```python
from build123d import *

# Parameters (mm, degrees)
F0_R     = 12.5
F1_DEPTH = 15


with BuildPart() as f1:
    # F0 (on Front) → F1 (new body)
    with BuildSketch(Plane.XZ):
        with BuildLine():
            ThreePointArc((-66.897273, -29.196363), (-41.384391, -23.525711), (-30, 0))
            ThreePointArc((-30, 0), (-41.384391, 23.525711), (-66.897273, 29.196363))
            ThreePointArc((-66.897273, 29.196363), (-90, 0), (-66.897273, -29.196363))
        make_face()
        with Locations((-60, 0)):
            Circle(F0_R, mode=Mode.SUBTRACT)
        with BuildLine():
            ThreePointArc((-66.897273, 29.196363), (-41.384391, 23.525711), (-30, 0))
            ThreePointArc((-30, 0), (-41.384391, -23.525711), (-66.897273, -29.196363))
            Line((-66.897273, -29.196363), (0, -45))
            Line((0, -45), (0, 45))
            Line((0, 45), (-66.897273, 29.196363))
        make_face()
    extrude(amount=F1_DEPTH)


solid = f1.part
```
CAD build for the part. Positions are in the model's coordinates, mm. Coordinates: 2 decimals unless noted, no trailing zeros. Write each loop counter-clockwise with the first axis right and the second up, starting at its lowest first coordinate (ties: lowest second). Pieces come first, ordered by that corner, then holes.
(1) Cut at A-A, the plane z = 0. List the corners of the cut face in (x, y).
(2) Flat gauge pins, fed straight in: pin 1 (6 mm diameter, centred on x = -30.5, y = -12, fed in from +Z); pin 2 (5 mm diameter, centred on x = -51.5, y = -3.5, fed in from +Z). Where does each tip first touch, or does it go through?
(3) Cut at C-C, the plane x = -60. List the corners of the cut face in (y, z), and give its area (3 significant figures).
(4) Two-plate mould, pull along Z, no slides. Class faces 1 (the face through (-72.488, -7.395, 0.55)), 2 (the face through (-33.917, -7.395, -36.988)), 3 (the face through (0, -7, -1)): +Z half, -Z half, draft (parallel to the pull), parting line (faces both ways), or undercut.
(5) Drill centre lines: probe 1 along Z at (x, y) = (-56.5, -10); probe 2 along X at (y, z) = (-1, -1); probe 3 along Z at (x, y) = (-60, -4.25). Where is each one in solid material? Low to high.
(6) Cut at B-B, the plane y = -6. List the corners of the cut face in (x, z).
(7) Cut at D-D, the plane x = -83. List the corners of the cut face in (y, z), and give its area (3 significant figures).
Geometry says:
1. outline: (-90, -15) - (-72.5, -15) - (-72.5, 0) - (-90, 0) - close; (-47.5, -15) - (0, -15) - (0, 0) - (-47.5, 0) - close
2. pin 1: stops at z = 38.5
2. pin 2: stops at z = 33.42
3. outline: (-15, -30.83) - (0, -30.83) - (0, -12.5) - (-15, -12.5) - close; (-15, 12.5) - (0, 12.5) - (0, 30.83) - (-15, 30.83) - close
3. area: 550 mm2
4. face 1: undercut
4. face 2: -Z half
4. face 3: draft
5. probe 1: z = -31.65 to -12, 12 to 31.65
5. probe 2: x = -89.98 to -72.46, -47.54 to 0
5. probe 3: z = -30.83 to -12.5, 12.5 to 30.83
6. outline: (-66.9, -29.2) - (0, -45) - (0, 45) - (-66.9, 29.2) arc R30 ccw to start; hole circle Ø25 at (-60, 0)
7. outline: (-15, -19.26) - (0, -19.26) - (0, 19.26) - (-15, 19.26) - close
7. area: 578 mm2
